```python
from build123d import *

# Parameters (mm, degrees)
PAD017_DEPTH          = 4
SKETCH037_R           = 5.1
POCKET015_DEPTH       = 5
POLARPATTERN010_COUNT = 4
SKETCH038_W           = 87.800004
SKETCH038_H           = 87.800004
POCKET016_DEPTH       = 5
SKETCH039_R           = 3
POCKET017_DEPTH       = 337.8512658378
POLARPATTERN011_COUNT = 4


with BuildPart() as part:
    # Sketch036 → Pad017 (new body)
    with BuildSketch(Plane.XY):
        with BuildLine():
            Line((-59, 52), (-59, -52))
            ThreePointArc((-59, -52), (-56.9497474683, -56.9497474683), (-52, -59))
            Line((-52, -59), (52, -59))
            ThreePointArc((52, -59), (56.9497474683, -56.9497474683), (59, -52))
            Line((59, -52), (59, 52))
            ThreePointArc((59, 52), (56.9497474683, 56.9497474683), (52, 59))
            Line((52, 59), (-52, 59))
            ThreePointArc((-52, 59), (-56.9497474683, 56.9497474683), (-59, 52))
        make_face()
    extrude(amount=PAD017_DEPTH)

    # Sketch037 → Pocket015 (cut)
    with BuildSketch(Plane.XY):
        with Locations((-43.9, 43.9)):
            Circle(SKETCH037_R)
    pocket015 = extrude(amount=POCKET015_DEPTH, mode=Mode.SUBTRACT)

    # PolarPattern010: Pocket015 ×4 about axis
    polarpattern010_axis = Axis((0, 0, 0), (0, 0, 1))
    for i in range(1, POLARPATTERN010_COUNT):
        add(pocket015.rotate(polarpattern010_axis, i * 360 / POLARPATTERN010_COUNT), mode=Mode.SUBTRACT)

    # Sketch038 (on Face5 of PolarPattern010) → Pocket016 (cut)
    with BuildSketch(Plane.XY.offset(4)):
        Rectangle(SKETCH038_W, SKETCH038_H)
    extrude(amount=-POCKET016_DEPTH, mode=Mode.SUBTRACT)

    # Sketch039 (on Face5 of Pocket016) → Pocket017 (cut, through all)
    with BuildSketch(Plane.XY.offset(4)):
        with Locations((-52, 52)):
            Circle(SKETCH039_R)
    pocket017 = extrude(amount=-POCKET017_DEPTH, mode=Mode.SUBTRACT)

    # PolarPattern011: Pocket017 ×4 about axis
    polarpattern011_axis = Axis((0, 0, 4), (0, 0, 1))
    for i in range(1, POLARPATTERN011_COUNT):
        add(pocket017.rotate(polarpattern011_axis, i * 360 / POLARPATTERN011_COUNT), mode=Mode.SUBTRACT)


with BuildPart() as part_1:
    # Body006 placement: moved
    add(part.part.moved(Location((0, 0, 42.1))))


solid = part_1.part
```
The model under review builds one solid part; all positions refer to its coordinate system, in mm. A direction names the side the tool comes from. Round coordinates to 2 decimals unless told otherwise and drop trailing zeros. Write each loop counter-clockwise with the first axis right and the second up, starting at its lowest first coordinate (ties: lowest second). Pieces come first, ordered by that corner, then holes.
(1) We need section C-C on z = 45.1. Give the boundary of the cut face in (x, y).
(2) Insertion check: pin 1 (13.5 mm diameter, centred on x = 43.9, y = 43.9, fed in from +Z). The pin has a flat end and moves straight along its axis. Give the tip position at first contact, or say it passes through.
(3) Machinability: for faces 1 (the flat face through (1, 59, 44)), 2 (the flat face through (43.9, -1, 44)), which of the approach directions +Z, -Z, +X, -X, +Y, -Y give a long, thin tool a straight path to every point of the face, cutting with its end or side? Answer none if there is none.
(4) We need section A-A on y = -34. Give the boundary of the cut face in (x, z).
(5) Mouldability with a two-part tool opening along X and no side actions: class faces 3 (the cylindrical face through (47.62, 47.39, 44.07)), 4 (the cylindrical face through (57, 56.9, 44.1)), 5 (the flat face through (-1, -59, 44)), 6 (the cylindrical face through (-57, -56.9, 44.1)) as +X half, -X half, draft (parallel to the pull), parting line (faces both ways), or undercut.
(6) We need section D-D on y = -50.5. Give the boundary of the cut face in (x, z), and give its area (3 significant figures).
(7) Wall thickness on L1, parallel to Y at x = 44, z = 44.6; L2, parallel to Y at x = -52, z = 45.05; L3, parallel to Y at x = -29, z = 43.4: over which ranges is each line inside the solid? List them lowest first.
Findings below:
1. outline: (-59, -52) arc R7 ccw to (-52, -59) - (52, -59) arc R7 ccw to (59, -52) - (59, 52) arc R7 ccw to (52, 59) - (-52, 59) arc R7 ccw to (-59, 52) - close; hole circle Ø6 at (-52, -52); hole circle Ø6 at (-52, 52); hole (-43.9, -38.8) arc R5.1 ccw (long way) to (-38.8, -43.9) - (38.8, -43.9) arc R5.1 ccw (long way) to (43.9, -38.8) - (43.9, 38.8) arc R5.1 ccw (long way) to (38.8, 43.9) - (-38.8, 43.9) arc R5.1 ccw (long way) to (-43.9, 38.8) - close; hole circle Ø6 at (52, -52); hole circle Ø6 at (52, 52)
2. pin 1: stops at z = 46.1
3. face 1: +Z, -Z, +X, -X, +Y
3. face 2: +Z, -Z
4. outline: (-59, 42.1) - (-43.9, 42.1) - (-43.9, 46.1) - (-59, 46.1) - close; (43.9, 42.1) - (59, 42.1) - (59, 46.1) - (43.9, 46.1) - close
5. face 3: undercut
5. face 4: +X half
5. face 5: draft
5. face 6: -X half
6. outline: (-59, 42.1) - (-54.6, 42.1) - (-54.6, 46.1) - (-59, 46.1) - close; (-49.4, 42.1) - (49.4, 42.1) - (49.4, 46.1) - (-49.4, 46.1) - close; (54.6, 42.1) - (59, 42.1) - (59, 46.1) - (54.6, 46.1) - close
6. area: 430 mm2
7. L1: y = -59 to -49, -38.8 to 38.8, 49 to 59
7. L2: y = -59 to -55, -49 to 49, 55 to 59
7. L3: y = -59 to -43.9, 43.9 to 59
